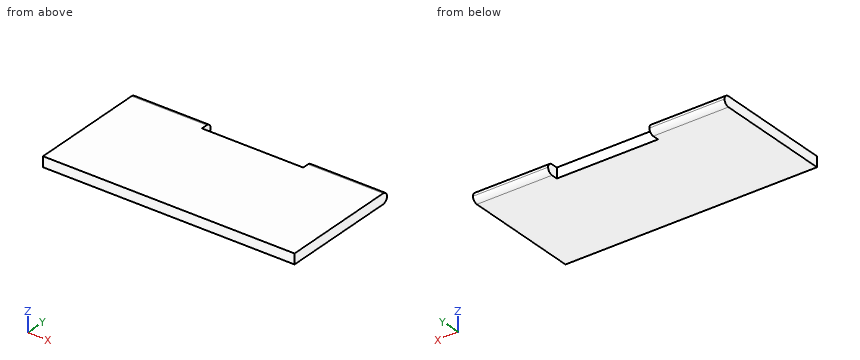
from build123d import *

# Parameters (mm, degrees)
SKETCH_1_W          = 308
SKETCH_1_H          = 150
EXTRUDE_1_DEPTH     = 12.5
FILLET_1_R          = 6.25
FILLET_2_R          = 6.25
CUT_EXTRUDE_1_DEPTH = 44


with BuildPart() as part:
    # 草图1 → 凸台-拉伸1 (new body)
    with BuildSketch(Plane.XY):
        with Locations((154, 75)):
            Rectangle(SKETCH_1_W, SKETCH_1_H)
    extrude(amount=EXTRUDE_1_DEPTH)

    # 圆角1
    fillet_1_edges = [part.edges().sort_by_distance(p)[0] for p in [
        (154, 150, 12.5),
    ]]
    fillet(fillet_1_edges, radius=FILLET_1_R)

    # 圆角2
    fillet_2_edges = [part.edges().sort_by_distance(p)[0] for p in [
        (154, 150, 0),
    ]]
    fillet(fillet_2_edges, radius=FILLET_2_R - 0.0001)  # a hair under: the kernel refuses the full size

    # 草图2 → 切除-拉伸1 (cut)
    with BuildSketch(Plane(origin=(0, 0, 0), x_dir=(-1, 0, 0), z_dir=(0, 0, -1))):
        Polygon((-154, 136), (-92, 136), (-92, 165.928579256), (-216, 165.928579256), (-216, 136), align=None)
    extrude(amount=-CUT_EXTRUDE_1_DEPTH, mode=Mode.SUBTRACT)


solid = part.part
Check sheet for the modelled part. Datum: model origin and axes. Units: mm. Coordinates: 2 decimals unless noted, no trailing zeros. Write each loop counter-clockwise with the first axis right and the second up, starting at its lowest first coordinate (ties: lowest second). Pieces come first, ordered by that corner, then holes.
Item 1: Cross-section at B-B on x = 162.5. Record the boundary of the cut face in (y, z), then the cut area to 3 significant figures.
Numbers:
outline: (0, 0) - (136, 0) - (136, 12.5) - (0, 12.5) - close
area: 1,700 mm2
Item 2: Cross-section at A-A on z = 10. Record the boundary of the cut face in (x, y), then the cut area to 3 significant figures.
Numbers:
outline: (0, 0) - (308, 0) - (308, 148.75) - (216, 148.75) - (216, 136) - (92, 136) - (92, 148.75) - (0, 148.75) - close
area: 44,200 mm2
Item 3: Scan lines: probe 1 along X at (y, z) = (141, 7.5); probe 2 along Y at (x, z) = (180, 4.5); probe 3 along Y at (x, z) = (80, 5.5). Record each from-to range of solid material in increasing order.
Numbers:
probe 1: x = 0 to 92, 216 to 308
probe 2: y = 0 to 136
probe 3: y = 0 to 149.95
Item 4: Depth check by flat-ended pin: pin 1 Ø6 at (y, z) = (62.5, 4) entering from -X; pin 2 Ø6 at (x, z) = (163.5, 8.5) entering from +Y. Enter the tip coordinate at first touch or a pass-through.
Numbers:
pin 1: stops at x = 0
pin 2: stops at y = 136
